Could you check a few things on this drawing? It's one solid part, dimensions in mm from its lowest x, y, z. A direction names the side the tool comes from. Give positions to 0.01 mm unless a question says otherwise; leave off trailing zeros. Order: outer loops, then holes, each group sorted by start corner. A loop starts at its lowest first (then second) coordinate and runs counter-clockwise, first axis right, second up.
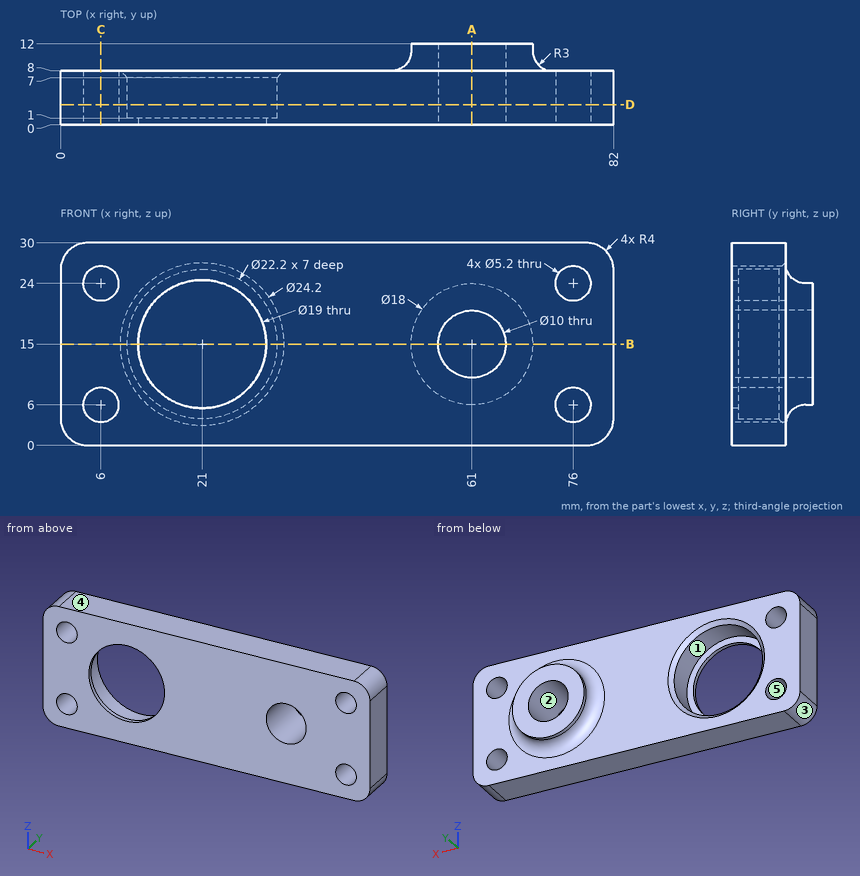
Item 1: Imagine slicing it at D-D on y = 3. List the corners of the cut face in (x, z) for me.
Findings:
outline: (0, 4) arc R4 ccw to (4, 0) - (78, 0) arc R4 ccw to (82, 4) - (82, 26) arc R4 ccw to (78, 30) - (4, 30) arc R4 ccw to (0, 26) - close; hole circle Ø5.2 at (6, 6); hole circle Ø5.2 at (6, 24); hole circle Ø22.2 at (21, 15); hole circle Ø10 at (61, 15); hole circle Ø5.2 at (76, 6); hole circle Ø5.2 at (76, 24)
Item 2: Imagine slicing it at C-C on x = 6. List the corners of the cut face in (y, z) for me.
Findings:
outline: (0, 0) - (8, 0) - (8, 3.4) - (0, 3.4) - close; (0, 8.6) - (8, 8.6) - (8, 21.4) - (0, 21.4) - close; (0, 26.6) - (8, 26.6) - (8, 30) - (0, 30) - close
Item 3: We'd pull the mould along X, two halves only. Please class the marked faces 3, 4 and 5: +X half, -X half, draft (parallel to the pull), parting line (faces both ways), or undercut.
Findings:
face 3: -X half
face 4: draft
face 5: undercut
Item 4: Imagine slicing it at B-B on z = 15. List the corners of the cut face in (x, y) for me, then the cut area to 3 significant figures.
Findings:
outline: (0, 0) - (11.5, 0) - (11.5, 1) - (9.9, 1) - (9.9, 7) - (8.9, 8) - (0, 8) - close; (30.5, 0) - (56, 0) - (56, 12) - (52, 12) - (52, 11) arc R3 cw to (49, 8) - (33.1, 8) - (32.1, 7) - (32.1, 1) - (30.5, 1) - close; (66, 0) - (82, 0) - (82, 8) - (73, 8) arc R3 cw to (70, 11) - (70, 12) - (66, 12) - close
area: 436 mm2
Item 5: Please list where these lines run through material, in increasing order: line 1 along X through (y, z) = (0.5, 15); line 2 along Z through (x, y) = (76, 4); line 3 along Z through (x, y) = (21, 0.2).
Findings:
line 1: x = 0 to 11.5, 30.5 to 56, 66 to 82
line 2: z = 0 to 3.4, 8.6 to 21.4, 26.6 to 30
line 3: z = 0 to 5.5, 24.5 to 30
Item 6: Imagine slicing it at A-A on x = 61. List the corners of the cut face in (y, z) for me.
Findings:
outline: (0, 0) - (8, 0) - (8, 3) arc R3 cw to (11, 6) - (12, 6) - (12, 10) - (0, 10) - close; (0, 20) - (12, 20) - (12, 24) - (11, 24) arc R3 cw to (8, 27) - (8, 30) - (0, 30) - close
Item 7: For pin 1 (2 mm diameter, centred on x = 65.5, z = 26, fed in from +Y), with a flat end and sliding along its axis, tell me the tip position at first contact or that it passes through.
Findings:
pin 1: stops at y = 8.21
Item 8: For the marked faces 1 and 2, which set-ups out of +Z, -Z, +X, -X, +Y, -Y let a thin tool reach every point of the face, with its end or its side?
Findings:
face 1: +Y
face 2: +Y, -Y
